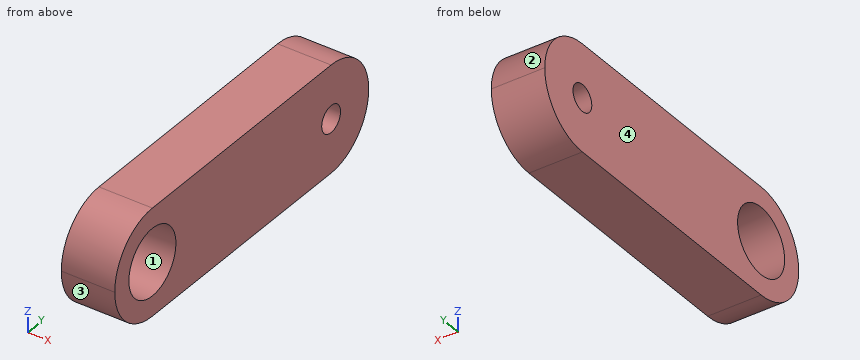
```python
from build123d import *

# Parameters (mm, degrees)
SKETCH1_W           = 8
SKETCH1_H           = 27
BOSS_EXTRUDE1_DEPTH = 4
SKETCH2_R           = 2.5
SKETCH2_R_2         = 1
CUT_EXTRUDE1_DEPTH  = 29.442925307
FILLET1_R           = 4


with BuildPart() as part:
    # Sketch1 → Boss-Extrude1 (new body)
    with BuildSketch(Plane(origin=(0, 0, 0), x_dir=(0, 0, -1), z_dir=(1, 0, 0))):
        with Locations((4, -13.5)):
            Rectangle(SKETCH1_W, SKETCH1_H)
    extrude(amount=BOSS_EXTRUDE1_DEPTH)

    # Sketch2 → Cut-Extrude1 (cut, through all)
    with BuildSketch(Plane(origin=(4, 0, 0), x_dir=(0, 0, -1), z_dir=(1, 0, 0))):
        with Locations((4, -23)):
            Circle(SKETCH2_R)
        with Locations((4, -4)):
            Circle(SKETCH2_R_2)
    extrude(amount=-CUT_EXTRUDE1_DEPTH, mode=Mode.SUBTRACT)

    # Fillet1
    fillet1_edges = [part.edges().sort_by_distance(p)[0] for p in [
        (2, -27, -8),
        (2, -27, 0),
        (2, 0, 0),
        (2, 0, -8),
    ]]
    fillet(fillet1_edges, radius=FILLET1_R - 0.0001)  # a hair under: the kernel refuses the full size


solid = part.part
```
CAD build for the part. Positions are in the model's coordinates, mm. Face numbers are marked on the shaded views. Round coordinates to 2 decimals unless told otherwise and drop trailing zeros. Write each loop counter-clockwise with the first axis right and the second up, starting at its lowest first coordinate (ties: lowest second). Pieces come first, ordered by that corner, then holes.
Item 1: Band-saw the part on B-B on z = -6. Write the cut outline in (x, y).
Filled in:
outline: (0, -26.46) - (4, -26.46) - (4, -24.5) - (0, -24.5) - close; (0, -21.5) - (4, -21.5) - (4, -0.54) - (0, -0.54) - close
Item 2: Band-saw the part on C-C on z = -2.5. Write the cut outline in (x, y).
Filled in:
outline: (0, -26.71) - (4, -26.71) - (4, -25) - (0, -25) - close; (0, -21) - (4, -21) - (4, -0.29) - (0, -0.29) - close
Item 3: Band-saw the part on D-D on z = -7.5. Write the cut outline in (x, y).
Filled in:
outline: (0, -24.94) - (4, -24.94) - (4, -2.06) - (0, -2.06) - close
Item 4: Drill centre lines: L1, parallel to Y at x = 1.95, z = -4; L2, parallel to Y at x = 1.9, z = -2.5; L3, parallel to Y at x = 3, z = -4.75. Where is each one in solid material? Low to high.
Filled in:
L1: y = -27 to -25.5, -20.5 to -5, -3 to 0
L2: y = -26.71 to -25, -21 to -0.29
L3: y = -26.93 to -25.38, -20.62 to -4.66, -3.34 to -0.07
Item 5: Band-saw the part on A-A on x = 1.6. Give the number of separate pieces and of enclosed holes in the cut face, then the cut area to 3 significant figures.
Filled in:
separate pieces: 1
enclosed holes: 2
area: 179 mm2
Item 6: Mould opens along Z. For the marked faces 1, 2, 3 and 4 say: released by +Z, released by -Z, zero draft, split by the parting line, or undercut.
Filled in:
face 1: undercut
face 2: released by +Z
face 3: released by -Z
face 4: zero draft
